The model under review builds one solid part; all positions refer to its coordinate system, in mm. A direction names the side the tool comes from. Give positions to 0.01 mm unless a question says otherwise; leave off trailing zeros. Loops run counter-clockwise (first coordinate to the right, second up) from the corner with the lowest first, then second, coordinate; pieces in that order, holes last. Notation, with made-up numbers: M 27,-33 L 50,-33 A7 ccw 50,-23 Z; hole C 26.5,-15 d6. An arc over 180 degrees is marked long. Put each result on its own line as item: value. Start each with the question number.
from build123d import *

# Parameters (mm, degrees)
SKETCH1_W           = 80
SKETCH1_H           = 50
BOSS_EXTRUDE1_DEPTH = 20
CUT_EXTRUDE1_DEPTH  = 20
SKETCH3_W           = 10
SKETCH3_H           = 30
CUT_EXTRUDE2_DEPTH  = 10
BOSS_EXTRUDE2_DEPTH = 10
SKETCH6_W           = 40
SKETCH6_H           = 20.022717562
BOSS_EXTRUDE3_DEPTH = 20
SKETCH7_W           = 20
SKETCH7_H           = 10
CUT_EXTRUDE3_DEPTH  = 10


with BuildPart() as part:
    # Sketch1 → Boss-Extrude1 (new body)
    with BuildSketch(Plane(origin=(0, 0, 0), x_dir=(1, 0, 0), z_dir=(0, 1, 0))):
        Rectangle(SKETCH1_W, SKETCH1_H)
    extrude(amount=BOSS_EXTRUDE1_DEPTH)

    # Sketch2 → Cut-Extrude1 (cut)
    with BuildSketch(Plane(origin=(0, 20, 0), x_dir=(1, 0, 0), z_dir=(0, 1, 0))):
        Polygon((-20, -25), (-20, -15), (-10, -15), (-10, -5), (10, -5), (10, -15), (30, -15), (30, -25), align=None)
    extrude(amount=-CUT_EXTRUDE1_DEPTH, mode=Mode.SUBTRACT)

    # Sketch3 → Cut-Extrude2 (cut)
    with BuildSketch(Plane(origin=(0, 20, 0), x_dir=(1, 0, 0), z_dir=(0, 1, 0))):
        with Locations((-35, -10)):
            Rectangle(SKETCH3_W, SKETCH3_H)
    extrude(amount=-CUT_EXTRUDE2_DEPTH, mode=Mode.SUBTRACT)

    # Sketch4 → Boss-Extrude2 (add)
    with BuildSketch(Plane(origin=(0, 20, 0), x_dir=(1, 0, 0), z_dir=(0, 1, 0))):
        Polygon((40, -25), (40, 25), (20, 25), (20, -15), (30, -15), (30, -25), align=None)
    extrude(amount=BOSS_EXTRUDE2_DEPTH)

    # Sketch6 → Boss-Extrude3 (add)
    with BuildSketch(Plane(origin=(0, 20, 0), x_dir=(1, 0, 0), z_dir=(0, 1, 0))):
        with Locations((0, 14.988641219)):
            Rectangle(SKETCH6_W, SKETCH6_H)
    extrude(amount=BOSS_EXTRUDE3_DEPTH)

    # Sketch7 → Cut-Extrude3 (cut)
    with BuildSketch(Plane(origin=(0, 40, 0), x_dir=(1, 0, 0), z_dir=(0, 1, 0))):
        with Locations((0, 9.977282438)):
            Rectangle(SKETCH7_W, SKETCH7_H)
    extrude(amount=-CUT_EXTRUDE3_DEPTH, mode=Mode.SUBTRACT)


solid = part.part
(1) To check wall thickness, follow L1, parallel to X at y = 18, z = 17; L2, parallel to Y at x = -17, z = 9; L3, parallel to X at y = 28.5, z = 4. State the ranges of each line that lie inside material, in increasing order. Write a range as [from, to].
(2) We need section C-C, the plane y = 17. Write out the cut boundary in (x, z), plus the area to 3 significant figures.
(3) We need section A-A, the plane z = 10.5. Write out the cut boundary in (x, y).
(4) For faces 1 (the flat face through (20, 35, -15)), 2 (the flat face through (-30, 15, 10)), 3 (the flat face through (0, 30, -10)), 4 (the flat face through (20, 11, 15)), list the 3-axis set-ups (+Z, -Z, +X, -X, +Y, -Y) from which the entire face can be reached by the end or side of a thin tool; tool diameter is ignored.
(5) We need section B-B, the plane x = 0.5. Write out the cut boundary in (y, z).
(6) Insertion check: pin 1 (16 mm diameter, centred on x = 9, y = 30.5, fed in from +Z); pin 2 (22 mm diameter, centred on x = -4.5, y = 11.5, fed in from +Z); pin 3 (1 mm diameter, centred on x = -16.5, z = 5, fed in from +Y). Each pin has a flat end and moves straight along its axis. Give the tip position at first contact, or say it passes through.
(7) We need section D-D, the plane z = -3. Write out the cut boundary in (x, y).
(8) Draft analysis for pull direction X (two halves, no side actions). For faces 5 (the flat face through (30, 15, 20)), 6 (the flat face through (30, 30, 0)), 7 (the flat face through (-40, 8, -5)), state which applies: +X half, -X half, draft (parallel to the pull), parting line (faces both ways), or undercut.
Check sheet entries:
1. L1: x = [-30, -20], [30, 40]
1. L2: y = [0, 20]
1. L3: x = [20, 40]
2. outline: M -40,-25 L 40,-25 L 40,25 L 30,25 L 30,15 L 10,15 L 10,5 L -10,5 L -10,15 L -20,15 L -20,25 L -30,25 L -30,-5 L -40,-5 Z
2. area: 3,000 mm²
3. outline: M -40,0 L -10,0 L -10,20 L -30,20 L -30,10 L -40,10 Z; M 10,0 L 40,0 L 40,30 L 20,30 L 20,20 L 10,20 Z
4. face 1: +Z, -Z, +X, +Y
4. face 2: +Z, -X, +Y
4. face 3: +Z, +Y
4. face 4: +Z, +Y, -Y
5. outline: M 0,-25 L 40,-25 L 40,-14.98 L 30,-14.98 L 30,-4.98 L 20,-4.98 L 20,5 L 0,5 Z
6. pin 1: stops at z = -4.98
6. pin 2: stops at z = 15
6. pin 3: stops at y = 20
7. outline: M -40,0 L 40,0 L 40,30 L 20,30 L 20,20 L -30,20 L -30,10 L -40,10 Z
8. face 5: undercut
8. face 6: draft
8. face 7: -X half
